Autodesk Inventor part; units mm, degrees
ref_plane "YZ Plane" through (0, 0, 0) normal (1, 0, 0) x (0, 1, 0)
ref_plane "XZ Plane" through (0, 0, 0) normal (0, 1, 0) x (-1, 0, 0)
ref_plane "XY Plane" through (0, 0, 0) normal (0, 0, 1) x (1, 0, 0)
sketch "Sketch1" plane through (0, 0, 0) normal (0, 0, 1) x (1, 0, 0)
  line L0 (0, 0) -> (38.1, 0)
  line L1 (38.1, 0) -> (38.1, 12.7)
  line L2 (38.1, 12.7) -> (0, 12.7)
  line L3 (0, 12.7) -> (0, 0)
  dimension "d0" = 38.1
  dimension "d1" = 12.7
extrude "Extrusion1" add sketch "Sketch1" along normal blind 3.175
sketch "Sketch2" plane through (0, 0, 3.175) normal (0, 0, 1) x (1, 0, 0)
  line L0 (38.1, 12.7) -> (0, 12.7)
  line L1 (0, 12.7) -> (0, 0)
  point P0 (6.35, 6.35)
  dimension "d4" = 6.35
  dimension "d5" = 6.35
hole "Hole1" at (6.35, 6.35, 3.175) direction (0, 0, -1) diameter 3.683 end through all
properties part number "RollerSquareBracket"
The listing builds one solid part. Answer for the finished solid, in the listing's coordinates (mm). Coordinates: 2 decimals unless noted, no trailing zeros. Order: outer loops, then holes, each group sorted by start corner. A loop starts at its lowest first (then second) coordinate and runs counter-clockwise, first axis right, second up.
Q1. A cutting plane is placed at C-C, the plane z = 0.65. Write down the section's boundary in (x, y).
Q2. For a pull along X with two mould halves and no side action, classify faces 1 (the face through (5.797, 4.594, 1.565)), 2 (the face through (38.1, 6, 2)), 3 (the face through (19, 6, 0)) as pulls with the +X half, pulls with the -X half, needs draft (parallel to the pull), parting line crosses it, or undercut.
Q3. Consider line 1 (X direction, y = 6.35, z = 1.1); line 2 (Y direction, x = 6.35, z = 2.1); line 3 (X direction, y = 4.75, z = 1.4). Determine where each line is inside the solid, lowest interval first.
Q4. A cutting plane is placed at A-A, the plane y = 6.35. Write down the section's boundary in (x, z) (1 decimal), and give its area (3 significant figures).
Q5. A cutting plane is placed at B-B, the plane x = 6.35. Write down the section's boundary in (y, z) (1 decimal).
Answers follow:
1. outline: (0, 0) - (38.1, 0) - (38.1, 12.7) - (0, 12.7) - close; hole circle Ø3.68 at (6.35, 6.35)
2. face 1: undercut
2. face 2: pulls with the +X half
2. face 3: needs draft
3. line 1: x = 0 to 4.51, 8.19 to 38.1
3. line 2: y = 0 to 4.51, 8.19 to 12.7
3. line 3: x = 0 to 5.44, 7.26 to 38.1
4. outline: (0, 0) - (4.5, 0) - (4.5, 3.2) - (0, 3.2) - close; (8.2, 0) - (38.1, 0) - (38.1, 3.2) - (8.2, 3.2) - close
4. area: 109 mm2
5. outline: (0, 0) - (4.5, 0) - (4.5, 3.2) - (0, 3.2) - close; (8.2, 0) - (12.7, 0) - (12.7, 3.2) - (8.2, 3.2) - close
